```python
from build123d import *

# Parameters (mm, degrees)
SKETCH1_R      = 3.175
EXTRUDE1_DEPTH = 41.671875
CHAMFER1_SIZE  = 0.635
EXTRUDE7_DEPTH = 59.117462213
FILLET1_R      = 1.5875


with BuildPart() as part:
    # Sketch1 → Extrude1 (new, symmetric)
    with BuildSketch(Plane.XY):
        Circle(SKETCH1_R)
    extrude(amount=EXTRUDE1_DEPTH, both=True)

    # Chamfer1
    chamfer1_edges = [part.edges().sort_by_distance(p)[0] for p in [
        (-3.175, 0, -41.671875),
        (-3.175, 0, 41.671875),
    ]]
    chamfer(chamfer1_edges, length=CHAMFER1_SIZE)

    # Sketch13 → Extrude7 (cut, through all)
    with BuildSketch(Plane.XY.offset(16.271875)):
        with BuildLine():
            Line((-1.5875, 2.749630657), (1.5875, 2.749630657))
            ThreePointArc((1.5875, 2.749630657), (0, 3.175), (-1.5875, 2.749630657))
        make_face()
    extrude(amount=EXTRUDE7_DEPTH, mode=Mode.SUBTRACT)

    # Fillet1
    # the kernel refuses this fillet: 1.5875 mm, written as the material it adds along each edge
    with BuildSketch(Plane(origin=(-5.55625, 2.749630657, 16.271875), x_dir=(0, 0, 1), z_dir=(1, 0, 0))) as fillet1_piece_1_section:
        with BuildLine():
            CenterArc((FILLET1_R, -FILLET1_R), FILLET1_R, 90, 90)
            Line((0, -FILLET1_R), (0, 0))
            Line((0, 0), (FILLET1_R, 0))
        make_face()
    fillet1_piece_1 = extrude(amount=11.1125, mode=Mode.PRIVATE)
    fillet1_piece_1 = fillet1_piece_1 & Plane(origin=(0, 0, 16.798205884), x_dir=(1, 0, 0), z_dir=(0, 0, 1)) * Cylinder(3.175, 29, mode=Mode.PRIVATE)
    add(fillet1_piece_1)


solid = part.part
```
CAD build for the part. Positions are in the model's coordinates, mm. A direction names the side the tool comes from. Round coordinates to 2 decimals unless told otherwise and drop trailing zeros. Write each loop counter-clockwise with the first axis right and the second up, starting at its lowest first coordinate (ties: lowest second). Pieces come first, ordered by that corner, then holes. Notation, with made-up numbers: (23, 50) - (44, 50) arc R11 ccw to (44, 70) - close; hole circle Ø9 at (59.5, 54). An arc over 180 degrees is marked (long way). Return JSON: item names as keys, results as strings. Group by question number.
Item 1: Flat gauge pins, fed straight in: pin 1 Ø1.6 at (x, z) = (0.5, 28) entering from +Y; pin 2 Ø3 at (x, z) = (-1, -15) entering from +Y (3 decimals); pin 3 Ø1.5 at (x, z) = (-2, -7.5) entering from +Y. Where does each tip first touch, or does it go through?
Item 2: Probe probe 1 along X at (y, z) = (0.25, 27.5); probe 2 along Y at (x, z) = (0.5, -1.5); probe 3 along Z at (x, y) = (-1.25, 2.5). List the from-to ranges inside material, lowest first.
Item 3: 3-axis set-ups, long thin cutter, end or side, ignore diameter. For faces 1 (the face through (0, 2.75, 29)), 2 (the face through (0, 0, 41.672)): which of +Z, -Z, +X, -X, +Y, -Y reach the whole face in a straight line?
Item 4: Band-saw the part on B-B on z = -31.5. List the corners of the cut face in (x, y) (3 decimals).
Resolved:
{
 "1": {"pin 1": "stops at y = 2.75", "pin 2": "stops at y = 3.175", "pin 3": "stops at y = 2.92"},
 "2": {"probe 1": "x = -3.17 to 3.17", "probe 2": "y = -3.14 to 3.14", "probe 3": "z = -41.42 to 41.42"},
 "3": {"face 1": "+Z, +X, -X, +Y", "face 2": "+Z, +X, -X, +Y, -Y"},
 "4": {"outline": "circle Ø6.35 at (0, 0)"}
}
